Geometry check sheet. Reference: the model listing, model coordinates, mm. A direction names the side the tool comes from. Give positions to 0.01 mm unless a question says otherwise; leave off trailing zeros. Order: outer loops, then holes, each group sorted by start corner. A loop starts at its lowest first (then second) coordinate and runs counter-clockwise, first axis right, second up.
Autodesk Inventor part; units mm, degrees
ref_plane "YZ Plane" through (0, 0, 0) normal (1, 0, 0) x (0, 1, 0)
ref_plane "XZ Plane" through (0, 0, 0) normal (0, 1, 0) x (-1, 0, 0)
ref_plane "XY Plane" through (0, 0, 0) normal (0, 0, 1) x (1, 0, 0)
sketch "Sketch1" plane through (0, 0, 0) normal (0, 0, 1) x (1, 0, 0)
  line L0 (-6, 10) -> (6, 10)
  line L1 (6, 10) -> (6, -10)
  line L2 (6, -10) -> (-6, -10)
  line L3 (-6, -10) -> (-6, 10)
  line L4 (-5.5, -21.5) -> (5.5, -21.5)
  line L5 (5.5, -21.5) -> (14.5, -12.5)
  line L6 (14.5, -12.5) -> (14.5, 4.5)
  line L7 (-5.5, -21.5) -> (-14.5, -12.5)
  line L8 (-14.5, -12.5) -> (-14.5, 4.5)
  line L9 (0, -32.2278) -> (0, 36.9858) construction
  circle A0 centre (0, 17) radius 7.5
  line L10 (-14.5, 4.5) -> (-6.731, 20.308)
  line L11 (14.5, 4.5) -> (6.731, 20.308)
  circle A1 centre (-12, 0) radius 1.1
  circle A2 centre (-12, -9) radius 1.1
  circle A3 centre (12, 0) radius 1.1
  circle A4 centre (12, -9) radius 1.1
  line L12 (7, 11) -> (-7, 11)
  line L13 (-7, 11) -> (-7, -11)
  line L14 (-7, -11) -> (7, -11)
  line L15 (7, -11) -> (7, 11)
  circle A5 centre (-12, 0) radius 2.6
  circle A6 centre (-12, -9) radius 2.6
  circle A7 centre (12, 0) radius 2.6
  circle A8 centre (12, -9) radius 2.6
  point P0 (0, 0)
  point P1 (0, -21.5)
  point P2 (0, 2.379)
  dimension "d0" = 12
  dimension "d1" = 20
  dimension "d2" = 10
  dimension "d3" = 6
  dimension "d4" = 11
  dimension "d5" = 21.5
  dimension "d6" = 0
  dimension "d7" = 135
  dimension "d8" = 135
  dimension "d9" = 14.5
  dimension "d10" = 14.5
  dimension "d11" = 15
  dimension "d12" = 38.5
  dimension "d13" = 17
  dimension "d14" = 17
  dimension "d15" = 2.2
  dimension "d18" = 9
  dimension "d21" = 24
  dimension "d24" = 12
  dimension "d25" = 0
  dimension "d30" = 1
  dimension "d34" = 1.5
  dimension "d35" = 1.5
  dimension "d36" = 1.5
  dimension "d37" = 1.5
extrude "Extrusion1" add sketch "Sketch1" along normal blind 1.5 contours L3 L2 L1 L0 A0 L12 L15 L14 L13 | A0 L12 L0 | L12 L13 L14 L15 A0 L11 L6 A7 A8 L5 L4 L7 L8 A6 A5 L10 | A0 L12 | A5 L8 | L6 A7 | A6 L8 | L6 A8 picked at (-14.0333, 0) picked at (14.0333, 0) picked at (-14.0333, -9) picked at (14.0333, -9)
extrude "Extrusion2" add sketch "Sketch1" along normal blind 10 contours L3 L2 L1 L0 A0 L12 L15 L14 L13 | A0 L12 L0
fillet "Fillet1" radius 2 14 edges at (-7, -11, 5.75) (7, -11, 5.75) (7, 11, 5.75) (5.5, -21.5, 0.75) (-5.5, -21.5, 0.75) (14.5, -12.5, 0.75) (-14.5, -12.5, 0.75) (14.5, 4.5, 0.75) (-7, 11, 5.75) (-14.5, 4.5, 0.75) (6, 10, 5) (-6, 10, 5) (-6, -10, 5) (6, -10, 5)
extrude "Extrusion3" [suppressed]
fillet "Fillet2" radius 1 8 edges at (7, 0, 1.5) (6.4142, 10.4142, 1.5) (0, 11, 1.5) (-6.4142, 10.4142, 1.5) (-7, 0, 1.5) (-6.4142, -10.4142, 1.5) (0, -11, 1.5) (6.4142, -10.4142, 1.5)
equation "\"d8\" = d7"
equation "\"d14\" = d13"
equation "\"d24\" = 0.5 * d21"
equation "\"d35\" = d34"
equation "\"d36\" = d34"
equation "\"d37\" = d34"
properties part number "skye_airspeed"
Item 1: Draft check along Y on faces 1 (the cylindrical face through (-6.4, 10.43, 6.3)), 2 (the cylindrical face through (-10.984, -8.579, 0.74)), 3 (the flat face through (-7, 2, 0)). Enter one of: released by +Y, released by -Y, zero draft, split by the parting line, or undercut.
Reported:
face 1: released by +Y
face 2: undercut
face 3: zero draft
Item 2: Sectioned sample at D-D (x = -11.75). Enter the section's corners in (y, z), and give its area (3 significant figures).
Reported:
outline: (-15.25, 0) - (-10.07, 0) - (-10.07, 1.5) - (-15.25, 1.5) - close; (-7.93, 0) - (-1.07, 0) - (-1.07, 1.5) - (-7.93, 1.5) - close; (1.07, 0) - (10.1, 0) - (10.1, 1.5) - (1.07, 1.5) - close
area: 31.6 mm2
Item 3: Scan lines: L1, parallel to Y at x = 12, z = 0.75; L2, parallel to X at y = -5.5, z = 8; L3, parallel to Y at x = -2.25, z = 3.25. Record each from-to range of solid material in increasing order.
Reported:
L1: y = -15 to -10.1, -7.9 to -1.1, 1.1 to 9.59
L2: x = -7 to -6, 6 to 7
L3: y = -11 to -10, 10 to 11
Item 4: Sectioned sample at C-C (y = 0). Enter the section's corners in (x, z).
Reported:
outline: (-14.5, 0) - (-13.1, 0) - (-13.1, 1.5) - (-14.5, 1.5) - close; (-10.9, 0) - (-6, 0) - (-6, 10) - (-7, 10) - (-7, 2.5) arc R1 cw to (-8, 1.5) - (-10.9, 1.5) - close; (6, 0) - (10.9, 0) - (10.9, 1.5) - (8, 1.5) arc R1 cw to (7, 2.5) - (7, 10) - (6, 10) - close; (13.1, 0) - (14.5, 0) - (14.5, 1.5) - (13.1, 1.5) - close
Item 5: Sectioned sample at A-A (z = 7.25). Enter the section's corners in (x, y).
Reported:
outline: (-7, -9) arc R2 ccw to (-5, -11) - (5, -11) arc R2 ccw to (7, -9) - (7, 9) arc R2 ccw to (5, 11) - (-5, 11) arc R2 ccw to (-7, 9) - close; hole (-6, -8) arc R2 ccw to (-4, -10) - (4, -10) arc R2 ccw to (6, -8) - (6, 8) arc R2 ccw to (4, 10) - (-4, 10) arc R2 ccw to (-6, 8) - close
Item 6: Gauge pin test, flat ends, axial feed: pin 1 (4 mm diameter, centred on x = 0, z = 5, fed in from +Y); pin 2 (2.5 mm diameter, centred on x = 12, y = 0, fed in from +Z); pin 3 (6 mm diameter, centred on x = -2.5, z = 6, fed in from -Y). Record the tip position at first contact, or that the pin passes through.
Reported:
pin 1: stops at y = 11
pin 2: stops at z = 1.5
pin 3: stops at y = -11
Item 7: Sectioned sample at B-B (y = -5). Enter the section's corners in (x, z).
Reported:
outline: (-14.5, 0) - (-6, 0) - (-6, 10) - (-7, 10) - (-7, 2.5) arc R1 cw to (-8, 1.5) - (-14.5, 1.5) - close; (6, 0) - (14.5, 0) - (14.5, 1.5) - (8, 1.5) arc R1 cw to (7, 2.5) - (7, 10) - (6, 10) - close
Item 8: Set-up check for faces 4 (the flat face through (-10, 2, 1.5)), 5 (the flat face through (0, -11, 6)), 6 (the flat face through (-6, 0, 5)), 7 (the cylindrical face through (6.43, 10.4, 6.3)): record each of +Z, -Z, +X, -X, +Y, -Y from which the full face is reachable in a straight line by a thin tool's end or side.
Reported:
face 4: +Z
face 5: +Z, +X, -X, -Y
face 6: +Z, -Z
face 7: +Z, +X, +Y
